The model under review builds one solid part; all positions refer to its coordinate system, in mm. A direction names the side the tool comes from. Round coordinates to 2 decimals unless told otherwise and drop trailing zeros. Order: outer loops, then holes, each group sorted by start corner. A loop starts at its lowest first (then second) coordinate and runs counter-clockwise, first axis right, second up.
Autodesk Inventor part; units mm, degrees
ref_plane "YZ Plane" through (0, 0, 0) normal (1, 0, 0) x (0, 1, 0)
ref_plane "XZ Plane" through (0, 0, 0) normal (0, 1, 0) x (-1, 0, 0)
ref_plane "XY Plane" through (0, 0, 0) normal (0, 0, 1) x (1, 0, 0)
sketch "Sketch1" plane through (0, 0, 0) normal (0, 1, 0) x (-1, 0, 0)
  line L0 (-7.0894, 4.7564) -> (8.1506, 4.7564)
  line L1 (8.1506, 4.7564) -> (8.1506, -5.7836)
  line L2 (8.1506, -5.7836) -> (-7.0894, -5.7836)
  line L3 (-7.0894, -5.7836) -> (-7.0894, 4.7564)
  circle A0 centre (5.2806, -0.5136) radius 1.77
  point P0 (0, 0)
  dimension "d0" = 10.54
  dimension "d1" = 15.24
  dimension "d2" = 3.54
  dimension "d3" = 2.87
  dimension "d4" = 5.27
extrude "Extrusion1" add sketch "Sketch1" along normal blind 1.32
sketch "Sketch2" plane through (0, 1.32, 0) normal (0, 1, 0) x (1, 0, 0)
  line L0 (7.0894, 5.7836) -> (-8.1506, 5.7836)
  line L1 (-2.0506, 5.7836) -> (7.0894, 5.7836)
  line L2 (7.0894, 5.7836) -> (7.0894, -4.7564)
  line L3 (7.0894, -4.7564) -> (-2.0506, -4.7564)
  line L4 (-2.0506, -4.7564) -> (-2.0506, 5.7836)
  point P0 (0, 0)
  dimension "d7" = 9.14
extrude "Extrusion2" add sketch "Sketch2" along normal blind 3.37
chamfer "Chamfer1" distance 1.4 distance2 3.175 1 edges at (-2.0506, 4.69, -0.5136) measured on face at (0.996, 4.69, -2.2703)
chamfer "Chamfer2" distance 0.5 distance2 3.175 1 edges at (3.2194, 4.69, -5.7836) measured on face at (1.9294, 4.69, -2.2703)
chamfer "Chamfer3" distance 0.5 distance2 3.175 1 edges at (3.2194, 4.69, 4.7564) measured on face at (1.9294, 4.69, -1.9369)
sketch "Sketch4" plane through (7.0894, 0, 4.7564) normal (1, 0, 0) x (0, 0, -1)
  line L0 (0, 0) -> (0, 1.515)
  line L1 (10.54, 0) -> (0, 0)
  line L2 (2.03, 3.47) -> (8.51, 3.47)
  line L3 (8.51, 3.47) -> (8.51, 2.92)
  line L4 (8.51, 2.92) -> (2.03, 2.92)
  line L5 (2.03, 2.92) -> (2.03, 3.47)
  line L6 (3.43, 3.47) -> (3.43, 2.92)
  line L7 (4.57, 3.47) -> (4.57, 2.92)
  line L8 (5.97, 3.47) -> (5.97, 2.92)
  line L9 (7.11, 3.47) -> (7.11, 2.92)
  point P0 (4.7564, 0)
  dimension "d19" = 0.55
  dimension "d20" = 2.92
  dimension "d21" = 6.48
  dimension "d22" = 1.4
  dimension "d23" = 1.4
  dimension "d24" = 1.4
  dimension "d25" = 2.54
  dimension "d26" = 4.57
extrude "Extrusion3" add sketch "Sketch4" along normal blind 14 contours L2 L6 L4 L5 | L2 L3 L4 L9
properties part number "Diode"
(1) Consider section B-B (z = 1). Write out the cut boundary in (x, y) (3 decimals).
Data:
outline: (-8.151, 0) - (-6.198, 0) - (-6.198, 1.32) - (-8.151, 1.32) - close; (-4.363, 0) - (7.089, 0) - (7.089, 4.69) - (-0.651, 4.69) - (-2.051, 1.515) - (-2.051, 1.32) - (-4.363, 1.32) - close
(2) Insertion check: pin 1 (5 mm diameter, centred on x = -6, z = -1.5, fed in from +Y); pin 2 (0.6 mm diameter, centred on x = 15.5, y = 3, fed in from +Z); pin 3 (1.5 mm diameter, centred on x = 12, y = 2, fed in from +Z); pin 4 (1.5 mm diameter, centred on x = 13, z = 2, fed in from +Y). Each pin has a flat end and moves straight along its axis. Give the tip position at first contact, or say it passes through.
Data:
pin 1: stops at y = 1.32
pin 2: stops at z = 2.73
pin 3: passes through
pin 4: stops at y = 3.47
(3) To check wall thickness, follow probe 1 along X at (y, z) = (0.7, -0.5); probe 2 along Y at (x, z) = (7.5, -2.5); probe 3 along Y at (x, z) = (-4.25, -2.5). State the ranges of each line that lie inside material, in increasing order.
Data:
probe 1: x = -8.15 to -7.05, -3.51 to 7.09
probe 2: y = 2.92 to 3.47
probe 3: y = 0 to 1.32
(4) Consider section C-C (y = 0.9). Write out the cut boundary in (x, z).
Data:
outline: (-8.15, -5.78) - (7.09, -5.78) - (7.09, 4.76) - (-8.15, 4.76) - close; hole circle Ø3.54 at (-5.28, -0.51)
(5) Consider section A-A (x = -4.5). Write out the cut boundary in (y, z), and give its area (3 significant figures).
Data:
outline: (0, -5.78) - (1.32, -5.78) - (1.32, -2.1) - (0, -2.1) - close; (0, 1.07) - (1.32, 1.07) - (1.32, 4.76) - (0, 4.76) - close
area: 9.72 mm2
(6) For faces 4 (the flat face through (14, 3.47, -3)), 5 (the flat face through (14, 2.92, -3)), 6 (the flat face through (0, 1, 4.756)), 7 (the flat face through (-4, 1.32, 1)), list the 3-axis set-ups (+Z, -Z, +X, -X, +Y, -Y) from which the entire face can be reached by the end or side of a thin tool; tool diameter is ignored.
Data:
face 4: +Z, -Z, +X, +Y
face 5: +Z, -Z, +X, -Y
face 6: +Z, +X, -X, +Y, -Y
face 7: +Z, -Z, -X, +Y
(7) Draft analysis for pull direction X (two halves, no side actions). For faces 1 (the flat face through (-8.151, 1, 0)), 2 (the flat face through (2.455, 3.08, -5.537)), 3 (the cylindrical face through (-3.512, 0.651, -0.591)), state which applies: pulls with the +X half, pulls with the -X half, needs draft (parallel to the pull), parting line crosses it, or undercut.
Data:
face 1: pulls with the -X half
face 2: needs draft
face 3: undercut
(8) Consider section D-D (z = -4.75). Write out the cut boundary in (x, y) (3 decimals).
Data:
outline: (-8.151, 0) - (7.089, 0) - (7.089, 4.69) - (-0.651, 4.69) - (-2.051, 1.515) - (-2.051, 1.32) - (-8.151, 1.32) - close
